Model file for the job. Use its own axes, mm. Face numbers are marked on the shaded views. Give positions to 0.01 mm unless a question says otherwise; leave off trailing zeros. Order: outer loops, then holes, each group sorted by start corner. A loop starts at its lowest first (then second) coordinate and runs counter-clockwise, first axis right, second up. Notation, with made-up numbers: (25.25, 28.5) - (30.25, 28.5) arc R23 ccw to (30.25, 66.5) - close; hole circle Ø6 at (-4, 81). An arc over 180 degrees is marked (long way). Use CSV: the item, a comma, the result in double quotes. Start each with the question number.
(1) Band-saw the part on D-D, the plane z = 51. Give the cut face in (x, y).
(2) Band-saw the part on B-B, the plane z = -56. Give the cut face in (x, y).
(3) Drop flat-ended pins along their axis: pin 1 Ø12 at (y, z) = (-2, 39.5) entering from -X; pin 2 Ø3 at (y, z) = (0, -14.5) entering from -X; pin 3 Ø1.5 at (y, z) = (20, 34) entering from -X. Give the stop position or say it passes through.
(4) Probe L1, parallel to Z at x = 10, y = 21.5; L2, parallel to Z at x = 18, y = -6; L3, parallel to X at y = 24, z = -14.5. List the from-to ranges inside material, lowest first.
(5) Band-saw the part on A-A, the plane x = -8. Give the cut face in (y, z), then the cut area to 3 significant figures.
(6) Band-saw the part on C-C, the plane y = 21. Count the separate pieces of the cut face and the enclosed holes in it, then the cut area to 3 significant figures.
(7) Pull direction Z, two halves, no side cores. Call the marked faces 1, 2 and 3: +Z half, -Z half, draft (parallel to the pull), parting line (faces both ways), or undercut.
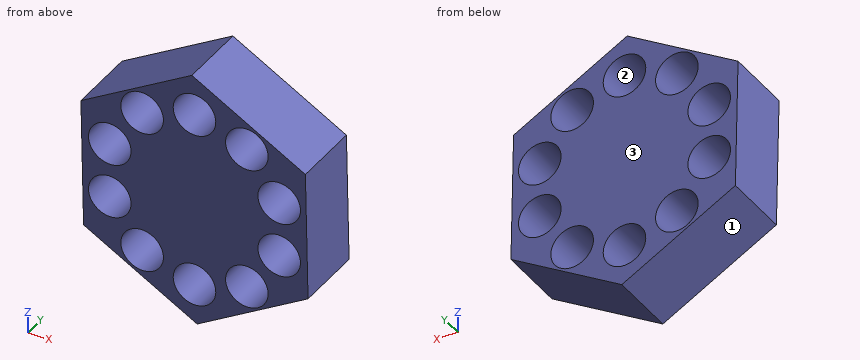
from build123d import *

# Parameters (mm, degrees)
BOSS_EXTRUDE1_DEPTH      = 27.178
BOSS_EXTRUDE1_DEPTH_BACK = 8.89
CUT_EXTRUDE1_REACH       = 100.213
SKETCH3_R                = 11.289480869
CIRPATTERN1_COUNT        = 10


with BuildPart() as part:
    # Sketch1 → Boss-Extrude1 (new, two sides: drawn at the far end of the back side and taken through both)
    with BuildSketch(Plane(origin=(0, 0, 0), x_dir=(1, 0, 0), z_dir=(0, 1, 0)).offset(-BOSS_EXTRUDE1_DEPTH_BACK)):
        Polygon((58.792489402, -35.575073205), (60.205161838, 33.128252771), (1.412672436, 68.703325976), (-58.792489402, 35.575073205), (-60.205161838, -33.128252771), (-1.412672436, -68.703325976), align=None)
    extrude(amount=BOSS_EXTRUDE1_DEPTH + BOSS_EXTRUDE1_DEPTH_BACK)

    # Sketch3 → Cut-Extrude1 (cut, up to next)
    with BuildSketch(Plane(origin=(0, 27.178, 0), x_dir=(1, 0, 0), z_dir=(0, 1, 0)), mode=Mode.PRIVATE) as cut_extrude1_sk1:
        with Locations(Location((0, -47.225969932, 0), (0, 0, 270))):
            Circle(SKETCH3_R)
    cut_extrude1_tool1 = extrude(cut_extrude1_sk1.sketch, amount=-CUT_EXTRUDE1_REACH, mode=Mode.PRIVATE) & part.part
    cut_extrude1 = cut_extrude1_tool1.solids().sort_by_distance((0, 27.178, 47.22597))[0]
    add(cut_extrude1, mode=Mode.SUBTRACT)

    # CirPattern1: Cut-Extrude1 ×10 about axis
    cirpattern1_axis = Axis((0, 0, 0), (0, 1, 0))
    for i in range(1, CIRPATTERN1_COUNT):
        add(cut_extrude1.rotate(cirpattern1_axis, i * 360 / CIRPATTERN1_COUNT), mode=Mode.SUBTRACT)


solid = part.part
Answer block:
1,outline,"(-30.67, -8.89) - (-10.64, -8.89) - (-10.64, 27.18) - (-30.67, 27.18) - close; (10.64, -8.89) - (30.76, -8.89) - (30.76, 27.18) - (10.64, 27.18) - close"
2,outline,"(-21.67, -8.89) - (-7.1, -8.89) - (-7.1, 27.18) - (-21.67, 27.18) - close; (7.1, -8.89) - (22.41, -8.89) - (22.41, 27.18) - (7.1, 27.18) - close"
3,pin 1,"stops at x = -59.59"
3,pin 2,"stops at x = -59.26"
3,pin 3,"stops at x = -60"
4,L1,"z = -63.51 to -52.47, -41.99 to 41.99, 52.47 to 62.42"
4,L2,"z = -58.67 to -43.88, -32.53 to 32.53, 43.88 to 58.02"
4,L3,"x = -59.23 to -56.2, -33.63 to 33.63, 56.2 to 59.82"
5,outline,"(-8.89, -63.52) - (27.18, -63.52) - (27.18, -55.19) - (-8.89, -55.19) - close; (-8.89, -39.26) - (27.18, -39.26) - (27.18, 39.26) - (-8.89, 39.26) - close; (-8.89, 55.19) - (27.18, 55.19) - (27.18, 64.72) - (-8.89, 64.72) - close"
5,area,"3,480 mm2"
6,separate pieces,"1"
6,enclosed holes,"10"
6,area,"8,260 mm2"
7,face 1,"-Z half"
7,face 2,"undercut"
7,face 3,"draft"
